Read the model definition and answer for the solid it produces. Units are mm, in the model's axes. Give positions to 0.01 mm unless a question says otherwise; leave off trailing zeros. Write each loop counter-clockwise with the first axis right and the second up, starting at its lowest first coordinate (ties: lowest second). Pieces come first, ordered by that corner, then holes. Notation, with made-up numbers: (87, 38.25) -> (91, 38.25) arc R16 ccw to (91, 51.25) -> close; hole circle Ø7 at (6, 18). An arc over 180 degrees is marked (long way). Write item = value, one per line.
from build123d import *

# Parameters (mm, degrees)
F1_DEPTH    = 152.4
F2_T1_DEPTH = 74.0210244843
F3_T1_DEPTH = 74.041
F4_W        = 14.6846622229
F4_H        = 6.4612496644
F5_DEPTH    = 12.7
F7_DEPTH    = 2.54
F9_DEPTH    = 2.54


# Not quite as in the source:
# - a fillet or chamfer that OpenCascade refuses, or shapes differently, is made with other operations: its cross-section is extruded or revolved along the edge and cut away or added


with BuildPart() as f1:
    # F0 (on Front) → F1 (new body)
    with BuildSketch(Plane.XZ):
        with BuildLine():
            Line((0, 19.05), (0, 6.35))
            ThreePointArc((0, 6.35), (1.8598719395, 1.8598719395), (6.35, 0))
            Line((6.35, 0), (95.25, 0))
            ThreePointArc((95.25, 0), (99.7401280605, 1.8598719395), (101.6, 6.35))
            Line((101.6, 6.35), (101.6, 19.05))
            ThreePointArc((101.6, 19.05), (99.7401280605, 23.5401280605), (95.25, 25.4))
            Line((95.25, 25.4), (6.35, 25.4))
            ThreePointArc((6.35, 25.4), (1.8598719395, 23.5401280605), (0, 19.05))
        make_face()
    extrude(amount=F1_DEPTH)

    # F2: fillet of radius 12.2642048969 on 1 edges, made by hand

    # F2_s2 → F2_t1 (cut)
    with BuildSketch(Plane.XY.offset(-24.3105122421)):
        with BuildLine():
            ThreePointArc((0, -140.1357951031), (3.5921024484, -148.8078975516), (12.2642048969, -152.4))
            Line((12.2642048969, -152.4), (0, -152.4))
            Line((0, -152.4), (0, -140.1357951031))
        make_face()
    extrude(amount=F2_T1_DEPTH, mode=Mode.SUBTRACT)

    # F3: fillet of radius 12.2682 on 1 edges, made by hand

    # F3_s2 → F3_t1 (cut)
    with BuildSketch(Plane.XY.offset(-24.3205)):
        with BuildLine():
            ThreePointArc((12.2682, 0), (3.593272587, -3.593272587), (0, -12.2682))
            Line((0, -12.2682), (0, 0))
            Line((0, 0), (12.2682, 0))
        make_face()
    extrude(amount=F3_T1_DEPTH, mode=Mode.SUBTRACT)

    # F4 (on face) → F5 (cut)
    with BuildSketch(Plane.XZ.offset(152.4)):
        with Locations((86.9044545794, 18.573864289)):
            Rectangle(F4_W, F4_H)
        with Locations((86.904451251, 6.8261355627)):
            Rectangle(F4_W, F4_H)
    extrude(amount=-F5_DEPTH, mode=Mode.SUBTRACT)

    # F6 (on face) → F7 (cut)
    with BuildSketch(Plane.XZ.offset(152.4)):
        Polygon((40.5169758041, 14.0975351255), (37.2149758041, 14.0975351255), (37.2149758041, 11.0495351255), (40.5169758041, 11.0495351255), (40.5169758041, 9.0060108787), (65.9169758041, 9.0060108787), (65.9169758041, 16.6260108787), (40.5169758041, 16.6260108787), align=None)
        Polygon((65.4089756118, 16.1180106864), (65.4089756118, 9.514011071), (41.0249759964, 9.514011071), (41.0249759964, 11.5575353178), (37.7229759964, 11.5575353178), (37.7229759964, 13.5895349332), (41.0249759964, 13.5895349332), (41.0249759964, 16.1180106864), align=None, mode=Mode.SUBTRACT)
    extrude(amount=-F7_DEPTH, mode=Mode.SUBTRACT)

    # F8 (on face) → F9 (cut)
    with BuildSketch(Plane.XZ.offset(152.4)):
        with BuildLine():
            Line((23.0576487401, 16.6260112998), (15.4376487401, 16.6260112998))
            ThreePointArc((15.4376487401, 16.6260112998), (14.539623128, 16.2540369119), (14.1676487401, 15.3560112998))
            Line((14.1676487401, 15.3560112998), (14.1676487401, 10.2760112998))
            ThreePointArc((14.1676487401, 10.2760112998), (14.539623128, 9.3779856877), (15.4376487401, 9.0060112998))
            Line((15.4376487401, 9.0060112998), (23.0576487401, 9.0060112998))
            ThreePointArc((23.0576487401, 9.0060112998), (23.9556743522, 9.3779856877), (24.3276487401, 10.2760112998))
            Line((24.3276487401, 10.2760112998), (24.3276487401, 15.3560112998))
            ThreePointArc((24.3276487401, 15.3560112998), (23.9556743522, 16.2540369119), (23.0576487401, 16.6260112998))
        make_face()
        with BuildLine():
            ThreePointArc((14.4295694742, 15.3560112998), (14.7248290552, 16.0688309847), (15.4376487401, 16.3640905657))
            Line((15.4376487401, 16.3640905657), (23.0576487401, 16.3640905657))
            ThreePointArc((23.0576487401, 16.3640905657), (23.770468425, 16.0688309847), (24.0657280061, 15.3560112998))
            Line((24.0657280061, 15.3560112998), (24.0657280061, 10.2760112998))
            ThreePointArc((24.0657280061, 10.2760112998), (23.770468425, 9.5631916149), (23.0576487401, 9.2679320338))
            Line((23.0576487401, 9.2679320338), (15.4376487401, 9.2679320338))
            ThreePointArc((15.4376487401, 9.2679320338), (14.7248290552, 9.5631916149), (14.4295694742, 10.2760112998))
            Line((14.4295694742, 10.2760112998), (14.4295694742, 15.3560112998))
        make_face(mode=Mode.SUBTRACT)
    extrude(amount=-F9_DEPTH, mode=Mode.SUBTRACT)


solid = f1.part
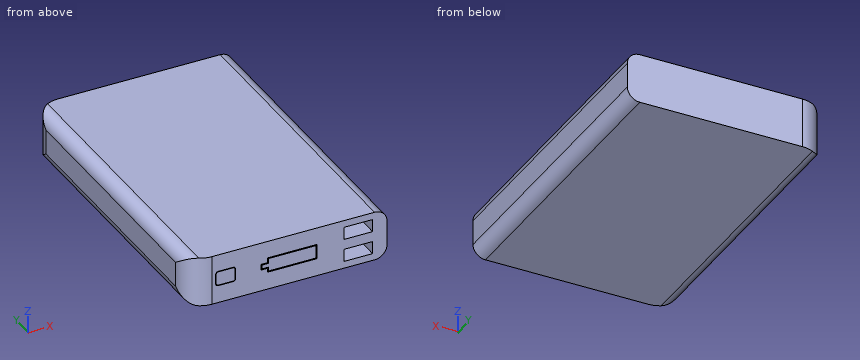
(1) The part is cut by section A-A on x = 88.5. Determine the outline of the cut face in (y, z).
Checks:
outline = (-152.4, 0) -> (0, 0) -> (0, 25.4) -> (-152.4, 25.4) -> (-152.4, 21.8) -> (-139.7, 21.8) -> (-139.7, 15.34) -> (-152.4, 15.34) -> (-152.4, 10.06) -> (-139.7, 10.06) -> (-139.7, 3.6) -> (-152.4, 3.6) -> close
(2) Consider L1, parallel to X at y = -7, z = 12.25; L2, parallel to X at y = -76.5, z = 20.75; L3, parallel to Z at x = 97, y = -63. Determine where each line is inside the solid, lowest interval first.
Checks:
L1 = 1.19 to 101.6
L2 = 0.23 to 101.37
L3 = 0.25 to 25.15
(3) The part is cut by section B-B on z = 23.5. Determine the outline of the cut face in (x, y), plus the area to 3 significant figures.
Checks:
outline = (1.82, -146.56) arc R12.26 ccw to (12.26, -152.4) -> (99.78, -152.4) -> (99.78, 0) -> (12.27, 0) arc R12.27 ccw to (1.82, -5.84) -> close
area = 14,900 mm²
(4) Given P1, Ø3, axis at x = 89, z = 5.5, coming from the -Y side; P2, Ø2, axis at y = -151, z = 12.5, coming from the -X side, each flat-ended and moving along its own axis, determine where each tip first touches the part or whether it passes through.
Checks:
P1 = -139.7
P2 = 4.98
